Print and shaded views of the part. All mm, measured from the part's lowest x, y and z. A direction names the side the tool comes from. Give positions to 0.01 mm unless a question says otherwise; leave off trailing zeros. Order: outer loops, then holes, each group sorted by start corner. A loop starts at its lowest first (then second) coordinate and runs counter-clockwise, first axis right, second up. Notation, with made-up numbers: (61, 23) - (118, 23) arc R7 ccw to (118, 30) - close; hole circle Ø9 at (36.25, 10). An arc over 180 degrees is marked (long way). Answer in a Markdown table with one row per item.
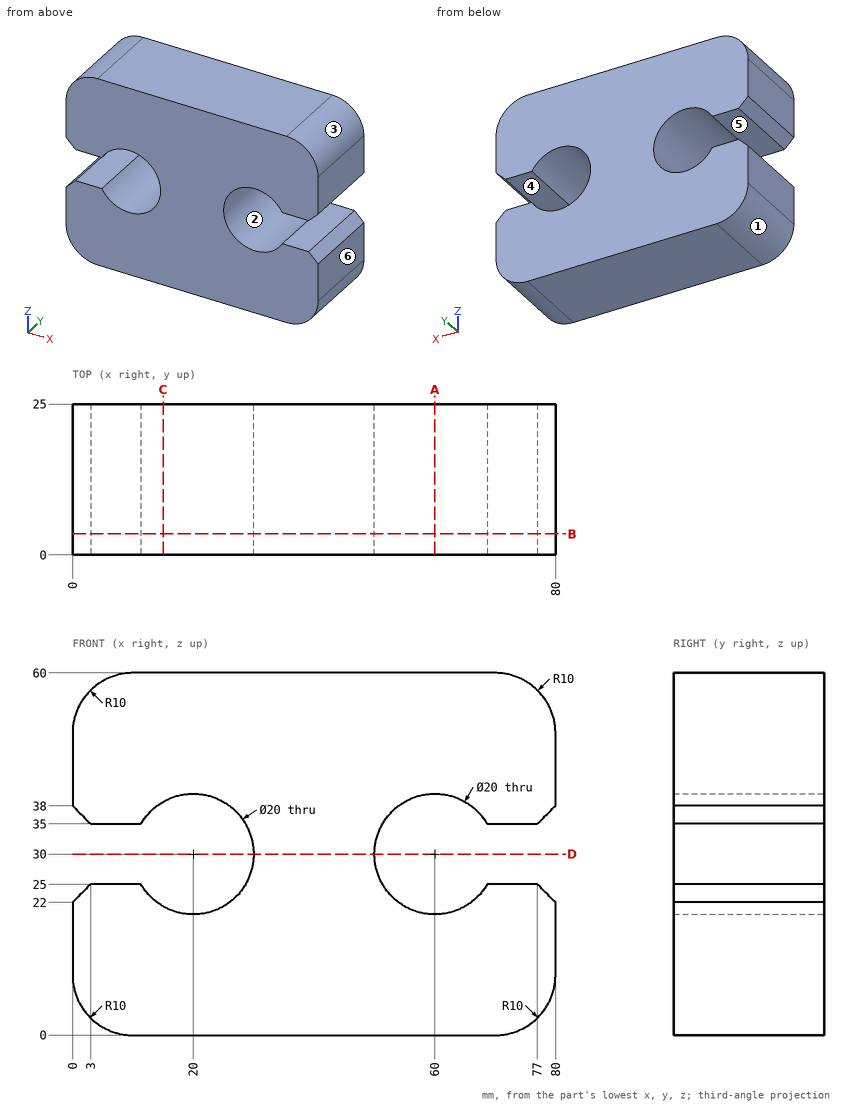
1. Probe line 1 (Z direction, x = 60, y = 19); line 2 (X direction, y = 18.25, z = 30); line 3 (Z direction, x = 57, y = 20.5). List the from-to ranges inside material, lowest first.
Check result:
| item | result |
|---|---|
| line 1 | z = 0 to 20, 40 to 60 |
| line 2 | x = 30 to 50 |
| line 3 | z = 0 to 20.46, 39.54 to 60 |
2. Cut at C-C on x = 15. Write the cut outline in (y, z), and give its area (3 significant figures).
Check result:
| item | result |
|---|---|
| outline | (0, 0) - (25, 0) - (25, 21.34) - (0, 21.34) - close; (0, 38.66) - (25, 38.66) - (25, 60) - (0, 60) - close |
| area | 1,070 mm² |
3. Two-plate mould, pull along Z, no slides. Class the marked faces 1, 2 and 3: +Z half, -Z half, draft (parallel to the pull), parting line (faces both ways), or undercut.
Check result:
| item | result |
|---|---|
| face 1 | -Z half |
| face 2 | undercut |
| face 3 | +Z half |
4. Which spindle directions (+Z, -Z, +X, -X, +Y, -Y) get a long thin tool onto all of the face, cutting with end or side? Do the marked faces 4, 5 and 6. Say none if no direction does.
Check result:
| item | result |
|---|---|
| face 4 | +X, +Y, -Y |
| face 5 | -X, +Y, -Y |
| face 6 | +Z, -Z, +X, +Y, -Y |
5. Cut at B-B on y = 3.5. Write the cut outline in (x, z), and give its area (3 significant figures).
Check result:
| item | result |
|---|---|
| outline | (0, 10) arc R10 ccw to (10, 0) - (70, 0) arc R10 ccw to (80, 10) - (80, 22) - (77, 25) - (68.66, 25) arc R10 cw (long way) to (68.66, 35) - (77, 35) - (80, 38) - (80, 50) arc R10 ccw to (70, 60) - (10, 60) arc R10 ccw to (0, 50) - (0, 38) - (3, 35) - (11.34, 35) arc R10 cw (long way) to (11.34, 25) - (3, 25) - (0, 22) - close |
| area | 3,860 mm² |
6. Cut at D-D on z = 30. Write the cut outline in (x, y).
Check result:
| item | result |
|---|---|
| outline | (30, 0) - (50, 0) - (50, 25) - (30, 25) - close |
7. Drop flat-ended pins along their axis: P1, Ø6.5, axis at x = 74, y = 6.5, coming from the -Z side; P2, Ø3, axis at y = 21.5, z = 30.5, coming from the -X side; P3, Ø2, axis at y = 15, z = 27.5, coming from the +X side. Give the stop position or say it passes through.
Check result:
| item | result |
|---|---|
| P1 | stops at z = 0.03 |
| P2 | stops at x = 29.8 |
| P3 | stops at x = 50.63 |
8. Cut at A-A on x = 60. Write the cut outline in (y, z), and give its area (3 significant figures).
Check result:
| item | result |
|---|---|
| outline | (0, 0) - (25, 0) - (25, 20) - (0, 20) - close; (0, 40) - (25, 40) - (25, 60) - (0, 60) - close |
| area | 1,000 mm² |
